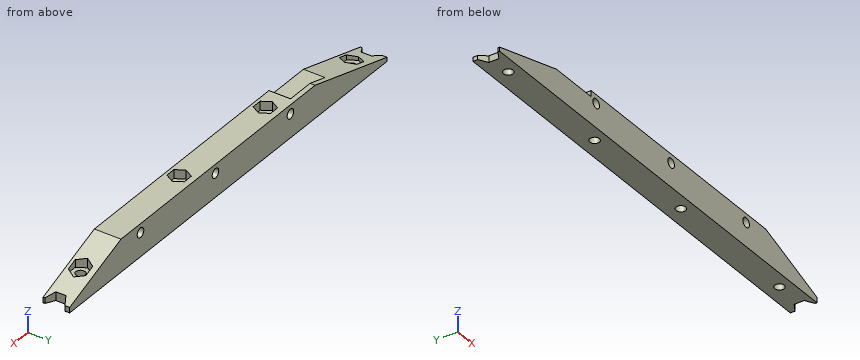
Autodesk Inventor part; units mm, degrees
ref_plane "YZ Plane" through (0, 0, 0) normal (1, 0, 0) x (0, 1, 0)
ref_plane "XZ Plane" through (0, 0, 0) normal (0, 1, 0) x (-1, 0, 0)
ref_plane "XY Plane" through (0, 0, 0) normal (0, 0, 1) x (1, 0, 0)
sketch "Sketch1" plane through (0, 0, 0) normal (0, 0, 1) x (1, 0, 0)
  line L0 (0, 0) -> (164.5, 0)
  line L1 (164.5, 0) -> (164.5, 9)
  line L2 (164.5, 9) -> (0, 9)
  line L3 (0, 9) -> (0, 0)
  circle A0 centre (57, 4) radius 1.6
  circle A1 centre (99, 4) radius 1.6
  circle A2 centre (159.5, 4) radius 1.6
  circle A3 centre (147, 4) radius 1.6
  circle A4 centre (15, 4) radius 1.6
  circle A5 centre (5, 4) radius 1.6
  dimension "d1" = 9
  dimension "d2" = 90
  dimension "d4" = 3.2
  dimension "d6" = 3.2
  dimension "d7" = 3.2
  dimension "d8" = 42
  dimension "d9" = 60.5
  dimension "d26" = 3.2
  dimension "d27" = 48
  dimension "d28" = 3.2
  dimension "d29" = 42
  dimension "d32" = 15
  dimension "d33" = 5
  dimension "d61" = 3.2
  dimension "d62" = 10
  dimension "d63" = 12.5
  dimension "d108" = 4
  dimension "d109" = 4
  dimension "d110" = 4
  dimension "d111" = 4
  dimension "d112" = 4
  dimension "d113" = 4
ref_plane "Work Plane2" through (0, 0, 0) normal (0, -1, 0) x (1, 0, 0)
sketch "Sketch2" plane through (0, 0, 0) normal (0, -1, 0) x (1, 0, 0)
  circle A0 centre (52, 8) radius 1.6
  circle A1 centre (125, 8) radius 1.6
  circle A2 centre (88.5, 8) radius 1.6
  point P0 (0, 0)
  point P1 (52, 0)
  dimension "d13" = 3.2
  dimension "d15" = 3.2
  dimension "d17" = 3.2
  dimension "d18" = 36.5
  dimension "d64" = 52
  dimension "d65" = 36.5
  dimension "d114" = 8
  dimension "d115" = 73
ref_plane "Work Plane1" through (0, 0, 11) normal (0, 0, 1) x (1, 0, 0)
extrude "klocek" add sketch "Sketch1" along normal blind 11
ref_plane "Work Plane3" through (0, 0, 0) normal (0, -1, 0) x (1, 0, 0)
extrude "prowadzenie osi" cut sketch "Sketch2" against normal up to next
ref_plane "Work Plane4" through (0, 0, 0) normal (0, -1, 0) x (1, 0, 0)
sketch "Sketch7" plane through (0, 0, 0) normal (0, -1, 0) x (1, 0, 0)
  line L0 (0, 11) -> (0, 0)
  line L1 (0, 11) -> (164.5, 11)
  line L2 (0, 11) -> (40, 11)
  line L3 (40, 11) -> (0, 0)
  point P0 (0, -1.8333)
  dimension "d86" = 11
  dimension "d87" = 40
sketch "Sketch8" plane through (0, 0, 0) normal (0, -1, 0) x (1, 0, 0)
  line L0 (164.5, 0) -> (164.5, 11)
  line L1 (164.5, 11) -> (164.5, 0)
  line L2 (164.5, 11) -> (0, 11)
  line L3 (164.5, 11) -> (134.5, 11)
  line L4 (134.5, 11) -> (164.5, 0)
  point P0 (0, 0)
  point P1 (40.8333, 11)
  dimension "d80" = 11
  dimension "d81" = 30
extrude "przedni skos" cut sketch "Sketch7" against normal up to next
extrude "tylni skos" cut sketch "Sketch8" against normal up to next
ref_plane "Work Plane7" through (0, 0, 11) normal (0, 0, 1) x (1, 0, 0)
sketch "Sketch5" plane through (0, 0, 11) normal (0, 0, 1) x (1, 0, 0)
  circle A0 centre (99, 4) radius 1.6
  line L0 (95.5936, 4) -> (97.2968, 6.95)
  line L1 (97.2968, 6.95) -> (100.7032, 6.95)
  line L2 (100.7032, 6.95) -> (102.4064, 4)
  line L3 (102.4064, 4) -> (100.7032, 1.05)
  line L4 (100.7032, 1.05) -> (97.2968, 1.05)
  line L5 (97.2968, 1.05) -> (95.5936, 4)
  circle A1 centre (57, 4) radius 1.6
  line L6 (60.4064, 4) -> (58.7032, 1.05)
  line L7 (58.7032, 1.05) -> (55.2968, 1.05)
  line L8 (55.2968, 1.05) -> (53.5936, 4)
  line L9 (53.5936, 4) -> (55.2968, 6.95)
  line L10 (55.2968, 6.95) -> (58.7032, 6.95)
  line L11 (58.7032, 6.95) -> (60.4064, 4)
  point P0 (119.5, 5)
  dimension "d98" = 5.9
  dimension "d100" = 5.9
extrude "hex insert middle" cut sketch "Sketch5" against normal blind 3
ref_plane "Work Plane6" through (0, 0, 11) normal (0, 0, 1) x (1, 0, 0)
sketch "Sketch9" plane through (0, 0, 11) normal (0, 0, 1) x (1, 0, 0)
  circle A0 centre (147, 4) radius 1.6
  line L0 (150.4064, 4) -> (148.7032, 1.05)
  line L1 (148.7032, 1.05) -> (145.2968, 1.05)
  line L2 (145.2968, 1.05) -> (143.5936, 4)
  line L3 (143.5936, 4) -> (145.2968, 6.95)
  line L4 (145.2968, 6.95) -> (148.7032, 6.95)
  line L5 (148.7032, 6.95) -> (150.4064, 4)
  point P0 (0, 0)
  point P1 (153, 5)
  dimension "d99" = 5.9
extrude "hex insert rear 1" cut sketch "Sketch9" against normal blind 6.5
ref_plane "Work Plane5" through (0, 0, 11) normal (0, 0, 1) x (1, 0, 0)
sketch "Sketch10" plane through (0, 0, 11) normal (0, 0, 1) x (1, 0, 0)
  circle A0 centre (159.5, 4) radius 1.6
  line L0 (162.45, 5.7032) -> (162.45, 2.2968)
  line L1 (162.45, 2.2968) -> (159.5, 0.5936)
  line L2 (159.5, 0.5936) -> (156.55, 2.2968)
  line L3 (156.55, 2.2968) -> (156.55, 5.7032)
  line L4 (156.55, 5.7032) -> (159.5, 7.4064)
  line L5 (159.5, 7.4064) -> (162.45, 5.7032)
  line L6 (164.5, 0) -> (134.5, 0)
  point P0 (0, 0)
  dimension "d118" = 5.9
extrude "hex insert rear 2" cut sketch "Sketch10" against normal up to next contours A0 | L0 L1 L2 L3 L4 L5
sketch "Sketch13" plane through (0, 0, 11) normal (0, 0, 1) x (1, 0, 0)
  line L0 (197.4, 0) -> (-32.9, 0)
  line L1 (7.95, 2.2968) -> (5, 0.5936)
  line L2 (5, 0.5936) -> (2.05, 2.2968)
  line L3 (2.05, 2.2968) -> (2.05, 5.7032)
  line L4 (2.05, 5.7032) -> (5, 7.4064)
  line L5 (5, 7.4064) -> (7.95, 5.7032)
  line L6 (7.95, 5.7032) -> (7.95, 2.2968)
  point P0 (0, 0)
  point P1 (5, 4)
  point P2 (5, 4)
  dimension "d117" = 5.9
extrude "hex insert front 1" cut sketch "Sketch13" against normal through all
sketch "Sketch16" plane through (0, 0, 11) normal (0, 0, 1) x (1, 0, 0)
  circle A0 centre (15, 4) radius 1.6
  line L0 (18.4064, 4) -> (16.7032, 1.05)
  line L1 (16.7032, 1.05) -> (13.2968, 1.05)
  line L2 (13.2968, 1.05) -> (11.5936, 4)
  line L3 (11.5936, 4) -> (13.2968, 6.95)
  line L4 (13.2968, 6.95) -> (16.7032, 6.95)
  line L5 (16.7032, 6.95) -> (18.4064, 4)
  point P0 (0, 0)
  dimension "d93" = 5.9
extrude "hex insert front 2" cut sketch "Sketch16" against normal blind 9
sketch "Sketch17" plane through (0, 0, 0) normal (0, 0, -1) x (-1, 0, 0)
  line L0 (0, 9) -> (0, 0)
  line L1 (0, 0) -> (-5, 0)
  line L2 (-5, 0) -> (-5, 10.0042)
  line L3 (-5, 10.0042) -> (0, 10.0042)
  line L4 (0, 10.0042) -> (0, 0)
  point P0 (-5, 7.4064)
extrude "ciecie przod" cut sketch "Sketch17" against normal up to next
sketch "Sketch18" plane through (40, 0, 11) normal (0, -1, 0) x (1, 0, 0)
  line L0 (9.5, 0) -> (9.5, -2)
  line L1 (9.5, -2) -> (-7.5, -2)
  line L2 (-7.5, -2) -> (-7.5, 0)
  line L3 (-7.5, 0) -> (9.5, 0)
  line L4 (94.5, 0) -> (0, 0)
  circle A0 centre (12, -3) radius 1.6
  line L5 (-35, -11) -> (124.5, -11)
  point P0 (-40, -11)
  dimension "d102" = 2
  dimension "d103" = 17
  dimension "d104" = 2.5
extrude "sensor linii" cut sketch "Sketch18" against normal blind 7.3 contours L0 L1 L2 L3
sketch "Sketch21" plane through (0, 0, 0) normal (0, 0, -1) x (-1, 0, 0)
  line L0 (-159.5, 8.9293) -> (-159.5, 0)
  line L1 (-164.5, 0) -> (-134.5, 0)
  line L2 (-159.5, 0) -> (-164.5, 0)
  line L3 (-164.5, 0) -> (-164.5, 9)
  line L4 (-164.5, 9) -> (-159.5, 9)
  line L5 (-159.5, 9) -> (-159.5, 8.9293)
  line L6 (-134.5, 9) -> (-164.5, 9)
  line L7 (-164.5, 9) -> (-164.5, 0)
  point P0 (0, 0)
extrude "ciecie tyl" cut sketch "Sketch21" against normal up to next
properties part number "wheel_support_v4_narrow_with_line_sensor_all_holes"
Model file for the job. Use its own axes, mm. Round coordinates to 2 decimals unless told otherwise and drop trailing zeros. Loops run counter-clockwise (first coordinate to the right, second up) from the corner with the lowest first, then second, coordinate; pieces in that order, holes last. Notation, with made-up numbers: (-40, 12) - (9, 12) arc R30 cw to (9, 48) - close; hole circle Ø4 at (45.25, 33). An arc over 180 degrees is marked (long way). Write each question's results on one line, items separated by ' | '.
(1) Saw through at C-C, the plane x = 15. List the corners of the cut face in (y, z) (3 decimals).
Answer below:
outline: (0, 0) - (2.4, 0) - (2.4, 2) - (1.05, 2) - (1.05, 4.125) - (0, 4.125) - close; (5.6, 0) - (9, 0) - (9, 4.125) - (6.95, 4.125) - (6.95, 2) - (5.6, 2) - close
(2) Saw through at B-B, the plane x = 136. List the corners of the cut face in (y, z).
Answer below:
outline: (0, 0) - (9, 0) - (9, 10.45) - (0, 10.45) - close
(3) Pin check, flat tips, straight feed: pin 1 (4 mm diameter, centred on y = 4, z = 2, fed in from -X); pin 2 (3 mm diameter, centred on x = 146.5, z = 5.5, fed in from -Y); pin 3 (2.5 mm diameter, centred on x = 57, y = 4, fed in from -Z); pin 4 (3.5 mm diameter, centred on x = 99, y = 4, fed in from +Z). Stop position of each tip, or through.
Answer below:
pin 1: stops at x = 7.44 | pin 2: stops at y = 0 | pin 3: passes through | pin 4: stops at z = 8
(4) Wall check: L1, parallel to Z at x = 88.5, y = 4; L2, parallel to Y at x = 15, z = 1.1; L3, parallel to Z at x = 45, y = 4. Give the ranges that are in metal, low to high.
Answer below:
L1: z = 0 to 6.4, 9.6 to 11 | L2: y = 0 to 2.4, 5.6 to 9 | L3: z = 0 to 9
(5) Saw through at A-A, the plane x = 99. List the corners of the cut face in (y, z), then the cut area to 3 significant figures.
Answer below:
outline: (0, 0) - (2.4, 0) - (2.4, 8) - (1.05, 8) - (1.05, 11) - (0, 11) - close; (5.6, 0) - (9, 0) - (9, 11) - (6.95, 11) - (6.95, 8) - (5.6, 8) - close | area: 55.7 mm^2
